Geometry: final body of the model. Coordinates: model frame, mm. A direction names the side the tool comes from. Give positions to 0.01 mm unless a question says otherwise; leave off trailing zeros. Write each loop counter-clockwise with the first axis right and the second up, starting at its lowest first coordinate (ties: lowest second). Pieces come first, ordered by that corner, then holes.
Q1. Reachability of faces 5 (the cylindrical face through (-7.26, -14.4, -23.04)), 6 (the cylindrical face through (8.46, -1.12, -20.4)) from +Z, -Z, +X, -X, +Y, -Y: full face, straight path, thin tool, end or side. Return the list, or none.
Q2. Line query: line 1 (Z direction, x = -4.5, y = -13); line 2 (X direction, y = -1.75, z = 0.5); line 3 (Z direction, x = -15, y = -1.5). Output: solid intervals per line, ascending.
Q3. Section C-C (y = -11). Return the cut outline in (x, z) (1 decimal).
Q4. Mould query, pull axis Y, two halves, no side actions, for faces 1 (the cylindrical face through (-20, -4.2, 2.6)), 2 (the flat face through (0, -15.24, 0)), 3 (the cylindrical face through (-7.26, -8.7, -23.04)), 4 (the cylindrical face through (-22.006, -11.668, -4.887)). Classes: +Y half, -Y half, draft (parallel to the pull), parting line (faces both ways), or undercut.
Q5. Pin query (flat end, axial travel): pin 1 Ø6 at (x, y) = (4, -12.5) entering from -Z; pin 2 Ø6 at (y, z) = (-4.5, -4) entering from -X; pin 3 Ø1 at (y, z) = (-3.5, -9.5) entering from +X. Return the tip coordinate at first contact, or that it passes through.
from build123d import *


with BuildPart() as part:
    # Sketch1 → Revolve1 (revolve)
    with BuildSketch(Plane.XY, mode=Mode.PRIVATE) as revolve1_sk:
        Polygon((-22.0853, 0), (-22.0853, -7.62), (-24.1554, -7.62), (-24.1554, -15.24), (0, -15.24), (0, 0), align=None)
    revolve(revolve1_sk.sketch.rotate(Axis((0, 0, 0), (0, 1, 0)), 270), axis=Axis((0, 0, 0), (0, 1, 0)))

    # Sketch7 → Groove for AS 568-132, O-Ring1 (revolve, cut)
    with BuildSketch(Plane(origin=(0, 0, 0), x_dir=(0, 0, -1), z_dir=(-1, 0, 0)), mode=Mode.PRIVATE) as groove_for_as_568_132_o_ring1_sk:
        with BuildLine():
            Line((22.774362441, 13.425029581), (24.6888, 13.592521165))
            Line((24.6888, 13.592521165), (24.6888, 9.701537998))
            Line((24.6888, 9.701537998), (22.774362441, 9.869029581))
            ThreePointArc((22.774362441, 9.869029581), (22.609231556, 9.950463122), (22.5425, 10.122063035))
            Line((22.5425, 10.122063035), (22.5425, 13.171996128))
            ThreePointArc((22.5425, 13.171996128), (22.609231556, 13.343596041), (22.774362441, 13.425029581))
        make_face()
    revolve(groove_for_as_568_132_o_ring1_sk.sketch.rotate(Axis((0, -50, 0), (0, 1, 0)), 180), axis=Axis((0, -50, 0), (0, 1, 0)), mode=Mode.SUBTRACT)

    # Sketch9 → Groove for AS 568-129, O-Ring1 (revolve, cut)
    with BuildSketch(Plane(origin=(0, 0, 0), x_dir=(0, 0, -1), z_dir=(-1, 0, 0))):
        with BuildLine():
            Line((20.399462441, 5.913991542), (22.3139, 6.081483126))
            Line((22.3139, 6.081483126), (22.3139, 2.190499959))
            Line((22.3139, 2.190499959), (20.399462441, 2.357991542))
            ThreePointArc((20.399462441, 2.357991542), (20.234331556, 2.439425083), (20.1676, 2.611024996))
            Line((20.1676, 2.611024996), (20.1676, 5.660958089))
            ThreePointArc((20.1676, 5.660958089), (20.234331556, 5.832558002), (20.399462441, 5.913991542))
        make_face()
    revolve(axis=Axis((0, -50, 0), (0, 1, 0)), mode=Mode.SUBTRACT)


solid = part.part
Computed:
1. face 5: +Y, -Y
1. face 6: +Y
2. line 1: z = -22.09 to 22.09
2. line 2: x = -22.08 to 22.08
2. line 3: z = -16.21 to 16.21
3. outline: circle Ø45.1 at (0, 0)
4. face 1: undercut
4. face 2: -Y half
4. face 3: draft
4. face 4: undercut
5. pin 1: stops at z = -24.13
5. pin 2: stops at x = -22.04
5. pin 3: stops at x = 18.05
